Source: CAD feature listing. Evaluate the final solid. Frame: model axes, mm. Give positions to 0.01 mm unless a question says otherwise; leave off trailing zeros. Write each loop counter-clockwise with the first axis right and the second up, starting at its lowest first coordinate (ties: lowest second). Pieces come first, ordered by that corner, then holes. Notation, with made-up numbers: M -32,-23 L -28,-23 A22 ccw -28,-9 Z; hole C 73.25,-5.5 d10. An arc over 180 degrees is marked long. Return JSON: item names as keys, results as strings.
```python
from build123d import *

# Parameters (mm, degrees)
F1_DEPTH = 25


with BuildPart() as f1:
    # F0 (on Front) → F1 (new body)
    with BuildSketch(Plane.XZ):
        with BuildLine():
            ThreePointArc((-5.160009, 0.057408), (7.6e-05, 4.339926), (5.160161, 0.057408))
            Line((5.160161, 0.057408), (10.223921, 0.057408))
            Line((10.223921, 0.057408), (10.223921, 11.362204))
            Line((10.223921, 11.362204), (-10.22377, 11.362204))
            Line((-10.22377, 11.362204), (-10.22377, 0.057408))
            Line((-10.22377, 0.057408), (-5.160009, 0.057408))
        make_face()
    extrude(amount=F1_DEPTH)


solid = f1.part
```
1) Draft query along X for faces 1 (the face through (-8, -12, 0.057)), 2 (the face through (-0.1, -12.32, 4.34)), 3 (the face through (-10.224, -12, 6)). Return one class per face: released by +X, released by -X, zero draft, split by the parting line, or undercut.
Numbers:
{"face 1": "zero draft", "face 2": "undercut", "face 3": "released by -X"}
2) Cut plane B-B, the plane y = -15. Return the cut outline in (x, z), then the cut area to 3 significant figures.
Numbers:
{"outline": "M -10.22,0.06 L -5.16,0.06 A5.25 cw 5.16,0.06 L 10.22,0.06 L 10.22,11.36 L -10.22,11.36 Z", "area": "198 mm²"}
3) Line query: line 1 (X direction, y = -9, z = 2); line 2 (X direction, y = -19, z = 3.5); line 3 (Z direction, x = -1.25, y = -5.5). Output: solid intervals per line, ascending. Write a range as [from, to].
Numbers:
{"line 1": "x = [-10.22, -4.37], [4.37, 10.22]", "line 2": "x = [-10.22, -2.85], [2.85, 10.22]", "line 3": "z = [4.19, 11.36]"}
4) Cut plane A-A, the plane z = 3. Return the cut outline in (x, y).
Numbers:
{"outline": "M -10.22,-25 L -3.5,-25 L -3.5,0 L -10.22,0 Z; M 3.5,-25 L 10.22,-25 L 10.22,0 L 3.5,0 Z"}
5) Cut plane D-D, the plane x = 3.5. Return the cut outline in (y, z).
Numbers:
{"outline": "M -25,3 L 0,3 L 0,11.36 L -25,11.36 Z"}
6) Cut plane C-C, the plane x = -3. Return the cut outline in (y, z), then the cut area to 3 significant figures.
Numbers:
{"outline": "M -25,3.4 L 0,3.4 L 0,11.36 L -25,11.36 Z", "area": "199 mm²"}
